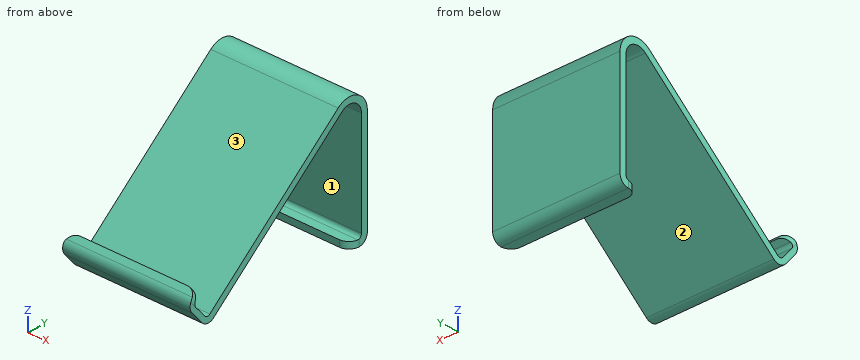
```python
from build123d import *

# Parameters (mm, degrees)
F1_DEPTH = 50
F2_R     = 7
F3_R     = 3
F4_R     = 7.99999


# Not quite as in the source:
# - a fillet or chamfer is up to 0.001 mm smaller than in the source, because OpenCascade refuses the exact size


with BuildPart() as f1:
    # F0 (on Right) → F1 (new body, symmetric)
    with BuildSketch(Plane.YZ):
        with BuildLine():
            Line((-152.5870774385, 20.6831999642), (-135.231811977, 0))
            Line((-135.231811977, 0), (-21.4278760969, 95.4928406235))
            ThreePointArc((-21.4278760969, 95.4928406235), (-10.7738173826, 96.8954740627), (-5, 87.8323961924))
            Line((-5, 87.8323961924), (-5, 5))
            Line((-5, 5), (-15, 5))
            Line((-15, 5), (-15, 0))
            Line((-15, 0), (0, 0))
            Line((0, 0), (0, 87.8323961924))
            ThreePointArc((0, 87.8323961924), (-8.6607260739, 101.4270129979), (-24.6418141453, 99.3230628391))
            Line((-24.6418141453, 99.3230628391), (-135.381572253, 6.4013726543))
            Line((-135.381572253, 6.4013726543), (-146.9517492273, 20.1901726305))
            Line((-146.9517492273, 20.1901726305), (-140.8233936824, 25.332473508))
            Line((-140.8233936824, 25.332473508), (-143.3945441211, 28.3966512805))
            Line((-143.3945441211, 28.3966512805), (-152.5870774385, 20.6831999642))
        make_face()
    extrude(amount=F1_DEPTH, both=True)

    # F2
    f2_edges = [f1.edges().sort_by_distance(p)[0] for p in [
        (0, -135.231812, 0),
        (0, -152.587077, 20.6832),
        (0, 0, 0),
    ]]
    fillet(f2_edges, radius=F2_R)

    # F3
    f3_edges = [f1.edges().sort_by_distance(p)[0] for p in [
        (0, -146.951749, 20.190173),
        (0, -135.381572, 6.401373),
        (0, -5, 5),
    ]]
    fillet(f3_edges, radius=F3_R)

    # F4 (radius 8 in the source; OpenCascade refuses exactly that, so slightly less here)
    f4_edges = [f1.edges().sort_by_distance(p)[0] for p in [
        (50, -142.108969, 26.864562),
        (-50, -142.108969, 26.864562),
        (50, -15, 2.5),
        (-50, -15, 2.5),
    ]]
    fillet(f4_edges, radius=F4_R)


solid = f1.part
```
Verification items for the finished model (mm, model axes). Face numbers are marked on the shaded views. Coordinates: 2 decimals unless noted, no trailing zeros. Loops run counter-clockwise (first coordinate to the right, second up) from the corner with the lowest first, then second, coordinate; pieces in that order, holes last. Notation, with made-up numbers: (12, -24.75) -> (33, -24.75) arc R29 ccw to (33, 6.25) -> close; hole circle Ø10 at (85, -25.5). An arc over 180 degrees is marked (long way). Answer in a Markdown table with one row per item.
1) Section check A-A (z = 37). Record the cut outline in (x, y).
The answers:
| item | result |
|---|---|
| outline | (-50, -98.92) -> (50, -98.92) -> (50, -91.14) -> (-50, -91.14) -> close; (-50, -5) -> (50, -5) -> (50, 0) -> (-50, 0) -> close |
2) Draft check along Z on the marked faces 1, 2 and 3. Enter one of: released by +Z, released by -Z, zero draft, split by the parting line, or undercut.
The answers:
| item | result |
|---|---|
| face 1 | undercut |
| face 2 | released by -Z |
| face 3 | released by +Z |
3) Scan lines: line 1 along Y through (x, z) = (28, 19.5); line 2 along Y through (x, z) = (23.5, 24); line 3 along Y through (x, z) = (-43, 92). Record each from-to range of solid material in increasing order. Write a range as from..to.
The answers:
| item | result |
|---|---|
| line 1 | y = -149.72..-145.71, -119.77..-111.99, -5..0 |
| line 2 | y = -148.34..-142.41, -114.41..-106.63, -5..0 |
| line 3 | y = -33.37..-25.59, -5.91..-0.59 |
4) Section check C-C (y = -58.5). Record the cut outline in (x, z), and give its area (3 significant figures).
The answers:
| item | result |
|---|---|
| outline | (-50, 64.39) -> (50, 64.39) -> (50, 70.91) -> (-50, 70.91) -> close |
| area | 653 mm2 |
5) Depth check by flat-ended pin: P1, Ø10, axis at x = -31.5, y = -123, coming from the +Z side; P2, Ø7.5, axis at x = 9.5, y = -12.5, coming from the +Z side; P3, Ø4, axis at x = 17, z = 1.5, coming from the -Y side; P4, Ø8, axis at x = -4, y = -86, coming from the +Z side. Enter the tip coordinate at first touch or a pass-through.
The answers:
| item | result |
|---|---|
| P1 | stops at z = 20.99 |
| P2 | stops at z = 102.83 |
| P3 | stops at y = -137.29 |
| P4 | stops at z = 51.19 |
6) Section check B-B (x = -36). Record the cut outline in (y, z).
The answers:
| item | result |
|---|---|
| outline | (-148.09, 15.32) -> (-139.73, 5.36) arc R7 ccw to (-129.87, 4.5) -> (-21.43, 95.49) arc R10 cw to (-5, 87.83) -> (-5, 8) arc R3 cw to (-8, 5) -> (-15, 5) -> (-15, 0) -> (-7, 0) arc R7 ccw to (0, 7) -> (0, 87.83) arc R15 ccw to (-24.64, 99.32) -> (-133.08, 8.33) arc R3 cw to (-137.31, 8.7) -> (-145.02, 17.89) arc R3 cw to (-144.65, 22.12) -> (-140.82, 25.33) -> (-143.39, 28.4) -> (-147.22, 25.18) arc R7 ccw to start |
